from build123d import *

# Parameters (mm, degrees)
SKETCH_1_W      = 100
SKETCH_1_H      = 10
SKETCH_1_R      = 1.75
SKETCH_1_W_2    = 20
EXTRUDE_1_DEPTH = 3


with BuildPart() as part:
    # 草图1 → 凸台-拉伸1 (new body)
    # profile 1 of 3: a face of its own
    with BuildSketch(Plane.XY):
        with Locations((50, 5)):
            Rectangle(SKETCH_1_W, SKETCH_1_H)
        with Locations((5, 5)):
            Circle(SKETCH_1_R, mode=Mode.SUBTRACT)
        with Locations((14, 5)):
            Circle(SKETCH_1_R, mode=Mode.SUBTRACT)
    # profile 2 of 3: a face of its own
    with BuildSketch(Plane.XY):
        with Locations((150, 5)):
            Rectangle(SKETCH_1_W, SKETCH_1_H)
        with Locations((195, 5)):
            Circle(SKETCH_1_R, mode=Mode.SUBTRACT)
    # profile 3 of 3: a face of its own
    with BuildSketch(Plane.XY):
        with Locations((210, 5)):
            Rectangle(SKETCH_1_W_2, SKETCH_1_H)
        with Locations((215, 5)):
            Circle(SKETCH_1_R, mode=Mode.SUBTRACT)
    extrude(amount=EXTRUDE_1_DEPTH)


solid = part.part
Here's how the part is built. I have some questions about the finished solid (model axes, mm). Coordinates: 2 decimals unless noted, no trailing zeros. Loops run counter-clockwise (first coordinate to the right, second up) from the corner with the lowest first, then second, coordinate; pieces in that order, holes last. Notation, with made-up numbers: (-36.75, 44.25) -> (-5.75, 44.25) arc R8 cw to (-5.75, 51.25) -> close; hole circle Ø2 at (70, -21.5). An arc over 180 degrees is marked (long way). Use one line per item in the form item = value. Start each with the question number.
(1) If we section it at B-B (z = 1.1): Please give me the cut outline in (x, y), then the cut area to 3 significant figures.
(2) If we section it at A-A (y = 5): Please give me the cut outline in (x, z).
(3) Please list where these lines run through material, in increasing order: line 1 along Y through (x, z) = (14, 0.9); line 2 along X through (y, z) = (3.5, 0.25); line 3 along X through (y, z) = (4, 1.5).
(4) We'd pull the mould along Y, two halves only. Please class faces 1 (the face through (213.25, 5.08, 1.48)), 2 (the face through (108, 5, 3)): pulls with the +Y half, pulls with the -Y half, needs draft (parallel to the pull), parting line crosses it, or undercut.
Verdict:
q1.outline = (0, 0) -> (220, 0) -> (220, 10) -> (0, 10) -> close; hole circle Ø3.5 at (5, 5); hole circle Ø3.5 at (14, 5); hole circle Ø3.5 at (195, 5); hole circle Ø3.5 at (215, 5)
q1.area = 2,160 mm²
q2.outline = (0, 0) -> (3.25, 0) -> (3.25, 3) -> (0, 3) -> close; (6.75, 0) -> (12.25, 0) -> (12.25, 3) -> (6.75, 3) -> close; (15.75, 0) -> (193.25, 0) -> (193.25, 3) -> (15.75, 3) -> close; (196.75, 0) -> (213.25, 0) -> (213.25, 3) -> (196.75, 3) -> close; (216.75, 0) -> (220, 0) -> (220, 3) -> (216.75, 3) -> close
q3.line_1 = 0 to 3.25, 6.75 to 10
q3.line_2 = 0 to 4.1, 5.9 to 13.1, 14.9 to 194.1, 195.9 to 214.1, 215.9 to 220
q3.line_3 = 0 to 3.56, 6.44 to 12.56, 15.44 to 193.56, 196.44 to 213.56, 216.44 to 220
q4.face_1 = undercut
q4.face_2 = needs draft
